from build123d import *

# Parameters (mm, degrees)
SKETCH1_W           = 88.9
SKETCH1_H           = 19.05
SKETCH1_R           = 9.525
BOSS_EXTRUDE1_DEPTH = 19.05
SKETCH1_3_W         = 101.6
SKETCH1_3_H         = 12.7
BOSS_EXTRUDE2_DEPTH = 38.1
SKETCH5_W           = 82.55
SKETCH5_H           = 19.05
SKETCH2_W           = 50.8
SKETCH2_H           = 9.525
SKETCH6_R           = 9.525
BOSS_EXTRUDE6_DEPTH = 6.35
SKETCH7_W           = 64.047051266
SKETCH7_H           = 6.35
BOSS_EXTRUDE7_DEPTH = 3.175


with BuildPart() as part:
    # Sketch1 → Boss-Extrude1 (new body)
    with BuildSketch(Plane.XY):
        with BuildLine():
            Line((0, 41.275), (0, 12.7))
            Line((0, 12.7), (101.6, 12.7))
            Line((101.6, 12.7), (101.6, 41.275))
            ThreePointArc((101.6, 41.275), (98.810192091, 48.010192091), (92.075, 50.8))
            Line((92.075, 50.8), (79.375, 50.8))
            Line((79.375, 50.8), (67.540629127, 72.591415535))
            ThreePointArc((67.540629127, 72.591415535), (50.8, 82.55), (34.059370873, 72.591415535))
            Line((34.059370873, 72.591415535), (22.225, 50.8))
            Line((22.225, 50.8), (9.525, 50.8))
            ThreePointArc((9.525, 50.8), (2.789807909, 48.010192091), (0, 41.275))
        make_face()
        with Locations((50.8, 34.925)):
            Rectangle(SKETCH1_W, SKETCH1_H, mode=Mode.SUBTRACT)
        with Locations((50.8, 63.5)):
            Circle(SKETCH1_R, mode=Mode.SUBTRACT)
        with Locations((50.8, 34.925)):
            Rectangle(SKETCH1_W, SKETCH1_H)
    extrude(amount=BOSS_EXTRUDE1_DEPTH)

    # Sketch1_3 → Boss-Extrude2 (add)
    with BuildSketch(Plane.XY):
        with Locations((50.8, 6.35)):
            Rectangle(SKETCH1_3_W, SKETCH1_3_H)
    extrude(amount=BOSS_EXTRUDE2_DEPTH)

    # Sketch5 → Loft1 section 0
    with BuildSketch(Plane.XY.offset(19.05)):
        with Locations((50.8, 34.925)):
            Rectangle(SKETCH5_W, SKETCH5_H)
    # Sketch2 → Loft1 section 1
    with BuildSketch(Plane.XY.offset(38.1)):
        with Locations((50.8, 30.1625)):
            Rectangle(SKETCH2_W, SKETCH2_H)
    loft()

    # Sketch6 → Boss-Extrude6 (add)
    with BuildSketch(Plane.XY.offset(19.05)):
        with BuildLine():
            Line((34.059370873, 72.591415535), (18.776474367, 44.45))
            Line((18.776474367, 44.45), (82.823525633, 44.45))
            Line((82.823525633, 44.45), (67.540629127, 72.591415535))
            ThreePointArc((67.540629127, 72.591415535), (50.8, 82.55), (34.059370873, 72.591415535))
        make_face()
        with Locations((50.8, 63.5)):
            Circle(SKETCH6_R, mode=Mode.SUBTRACT)
    extrude(amount=BOSS_EXTRUDE6_DEPTH)

    # Sketch7 → Boss-Extrude7 (add)
    with BuildSketch(Plane.XZ.offset(-44.45)):
        with Locations((50.8, 22.225)):
            Rectangle(SKETCH7_W, SKETCH7_H)
    extrude(amount=BOSS_EXTRUDE7_DEPTH)


solid = part.part
Check sheet for the modelled part. Datum: model origin and axes. Units: mm. A direction names the side the tool comes from. Give positions to 0.01 mm unless a question says otherwise; leave off trailing zeros. Write each loop counter-clockwise with the first axis right and the second up, starting at its lowest first coordinate (ties: lowest second). Pieces come first, ordered by that corner, then holes. Notation, with made-up numbers: (1, 24.25) -> (9, 24.25) arc R27 cw to (9, 50.25) -> close; hole circle Ø8 at (28.25, 51). An arc over 180 degrees is marked (long way). One line per item, written item: value. Start each with the question number.
Item 1: Tool access check on faces 5 (the flat face through (86, 50.8, 9)), 6 (the flat face through (50, 24, 19.05)), 7 (the flat face through (50, 53, 25.4)), 8 (the flat face through (82.824, 44, 24)). Record the directions out of +Z, -Z, +X, -X, +Y, -Y that give a thin tool (end or side, any length) a straight path to the whole face; none if there is none.
Item 2: Draft check along Y on faces 1 (the flat face through (50, 12.7, 28)), 2 (the flat face through (18.776, 44, 24)), 3 (the cylindrical face through (55.92, 71.53, 12.52)), 4 (the flat face through (16, 50.8, 9)). Enter one of: +Y half, -Y half, draft (parallel to the pull), parting line (faces both ways), or undercut.
Item 3: Section check C-C on x = 94. Record the cut outline in (y, z).
Item 4: Section check B-B on y = 19.5. Record the cut outline in (x, z), then the cut area to 3 significant figures.
Item 5: Section check A-A on y = 63.5. Record the cut outline in (x, z) (3 decimals).
Item 6: Gauge pin test, flat ends, axial feed: pin 1 (6.5 mm diameter, centred on x = 86.5, z = 11, fed in from +Y); pin 2 (12.5 mm diameter, centred on x = 39, y = 56, fed in from +Z); pin 3 (1.6 mm diameter, centred on y = 43.5, z = 21.5, fed in from +X). Record the tip position at first contact, or that the pin passes through.
Item 7: Material ranges on probe 1 along Y at (x, z) = (50.8, 6.25) (3 decimals); probe 2 along Z at (x, y) = (6, 16); probe 3 along Z at (x, y) = (41, 68.5), recorded low to high. Write a range as from..to.
Results list:
1. face 5: +Z, -Z, +X, +Y
1. face 6: +Z
1. face 7: +Z, +X, -X, +Y
1. face 8: +Z, +X, +Y
2. face 1: undercut
2. face 2: draft
2. face 3: undercut
2. face 4: +Y half
3. outline: (0, 0) -> (50.6, 0) -> (50.6, 19.05) -> (12.7, 19.05) -> (12.7, 38.1) -> (0, 38.1) -> close
4. outline: (0, 0) -> (101.6, 0) -> (101.6, 19.05) -> (0, 19.05) -> close
4. area: 1,940 mm²
5. outline: (29.122, 0) -> (41.275, 0) -> (41.275, 25.4) -> (29.122, 25.4) -> close; (60.325, 0) -> (72.478, 0) -> (72.478, 25.4) -> (60.325, 25.4) -> close
6. pin 1: y = 50.8
6. pin 2: z = 25.4
6. pin 3: x = 90.7
7. probe 1: 0..53.975, 73.025..82.55
7. probe 2: 0..19.05
7. probe 3: 0..25.4
